The model under review builds one solid part; all positions refer to its coordinate system, in mm. A direction names the side the tool comes from. Coordinates: 2 decimals unless noted, no trailing zeros. Order: outer loops, then holes, each group sorted by start corner. A loop starts at its lowest first (then second) coordinate and runs counter-clockwise, first axis right, second up. Notation, with made-up numbers: (-23, 21.25) - (-9, 21.25) arc R28 cw to (-9, 48.25) - close; hole circle Ø1 at (5, 74.5). An arc over 180 degrees is marked (long way). Answer in a Markdown table with one row per item.
Autodesk Inventor part; units mm, degrees
ref_plane "YZ Plane" through (0, 0, 0) normal (1, 0, 0) x (0, 1, 0)
ref_plane "XZ Plane" through (0, 0, 0) normal (0, 1, 0) x (-1, 0, 0)
ref_plane "XY Plane" through (0, 0, 0) normal (0, 0, 1) x (1, 0, 0)
sketch "Esboço1" plane through (0, 0, 0) normal (1, 0, 0) x (0, 1, 0)
  line L0 (-1.6, 0) -> (9.6, 0) construction
  line L1 (0, -42) -> (0, 42) construction
  line L2 (8, 30) -> (0, 30)
  line L3 (0, 30) -> (0, -30)
  line L4 (0, -30) -> (8, -30)
  line L5 (8, -30) -> (8, 30)
  line L6 (5.1132, 30) -> (8, 25)
  point P0 (0, 0)
  dimension "d0" = 16
  dimension "d1" = 60
  dimension "d2" = 5
  dimension "d3" = 30
revolve "Revolução1" add sketch "Esboço1" angle 360 about axis through (0, 0, 30) along (0, 0, -1) contours L6 L5 L4 L3 L2
fillet "Arredondamento1" radius 1 2 edges at (0, -5.1132, 30) (0, -8, 25)
sketch "Esboço2" plane through (0, 0, -30) normal (0, 0, -1) x (-1, 0, 0)
  circle A0 centre (0, 0) radius 8
hole "Furo1" at (0, 0, -30) direction (0, 0, 1) diameter 4.917 depth 20 tip angle 118
properties material "Aço SAE 1045"
Item 1: Clearance check with flat-ended pins moving along their axes: pin 1 Ø1.5 at (x, z) = (1, 18.5) entering from -Y; pin 2 Ø8 at (y, z) = (4.5, 19) entering from -X; pin 3 Ø1.5 at (x, z) = (2.5, -10.5) entering from +Y; pin 4 Ø8 at (y, z) = (2.5, 8.5) entering from +X. State where each tip first meets the part, or that it passes through.
Check values:
| item | result |
|---|---|
| pin 1 | y = -8 |
| pin 2 | x = -7.98 |
| pin 3 | y = 7.81 |
| pin 4 | x = 8 |
Item 2: To check wall thickness, follow line 1 (Y direction, x = 0, z = -23); line 2 (Y direction, x = -0.5, z = -25.5). State the ranges of each line that lie inside material, in increasing order. Write a range as from..to.
Check values:
| item | result |
|---|---|
| line 1 | -8..-2.46, 2.46..8 |
| line 2 | -7.98..-2.41, 2.41..7.98 |
Item 3: We need section A-A, the plane z = -15. Write out the cut boundary in (x, y), then the cut area to 3 significant figures.
Check values:
| item | result |
|---|---|
| outline | circle Ø16 at (0, 0); hole circle Ø4.92 at (0, 0) |
| area | 182 mm^2 |
Item 4: Tool access review of faces 1 (the face through (-0.738, 2.345, -19.86)), 2 (the face through (0, 0, 30)): name each direction out of +Z, -Z, +X, -X, +Y, -Y from which nothing blocks a thin tool from reaching the whole face with its end or side.
Check values:
| item | result |
|---|---|
| face 1 | -Z |
| face 2 | +Z, +X, -X, +Y, -Y |
Item 5: We need section B-B, the plane z = 10. Write out the cut boundary in (x, y).
Check values:
| item | result |
|---|---|
| outline | circle Ø16 at (0, 0) |
